Build history of the part. All positions in model axes, mm. Face numbers are marked on the shaded views. A direction names the side the tool comes from. Give positions to 0.01 mm unless a question says otherwise; leave off trailing zeros. Order: outer loops, then holes, each group sorted by start corner. A loop starts at its lowest first (then second) coordinate and runs counter-clockwise, first axis right, second up. Notation, with made-up numbers: (24, 44) -> (53, 44) arc R15 cw to (53, 65) -> close; hole circle Ø10 at (53, 45). An arc over 180 degrees is marked (long way). One line per item, written item: value. Start each with the question number.
(1) Pin check, flat tip, straight feed: pin 1 (2.5 mm diameter, centred on x = 10, z = 21, fed in from +Y). Stop position of the tip, or through.
(2) Two-plate mould, pull along X, no slides. Class the marked faces 1, 2, 3 and 4: +X half, -X half, draft (parallel to the pull), parting line (faces both ways), or undercut.
(3) Saw through at C-C on y = -10.25. Give the cut face in (x, z), plus the area to 3 significant figures.
(4) Saw through at A-A on y = -26.5. Give the cut face in (x, z), plus the area to 3 significant figures.
(5) Saw through at B-B on x = -4. Give the cut face in (y, z).
(6) Probe line 1 (Z direction, x = 13, y = -20.25); line 2 (Z direction, x = -8, y = -2.25); line 3 (Y direction, x = 16, z = 17.75). List the from-to ranges inside material, lowest first.
(7) Which spindle directions (+Z, -Z, +X, -X, +Y, -Y) get a long thin tool onto all of the face, cutting with end or side? Do the marked faces 5, 6 and 7. Say none if no direction does.
(8) Saw through at D-D on z = 22.25. Give the cut face in (x, y).
```python
from build123d import *

# Parameters (mm, degrees)
BOSS_EXTRUDE1_DEPTH         = 20.5
FILLET1_R                   = 2
M6_TAPPED_HOLE1_D           = 5
M6_TAPPED_HOLE1_DEPTH       = 17
M6_TAPPED_HOLE1_CSINK_D     = 6.05
M6_TAPPED_HOLE1_CSINK_ANGLE = 90
M6_TAPPED_HOLE1_TIP         = 1.502151548
FILLET2_R                   = 2


with BuildPart() as part:
    # Sketch1 → Boss-Extrude1 (new, symmetric)
    with BuildSketch(Plane(origin=(0, 0, 0), x_dir=(0, 0, -1), z_dir=(1, 0, 0))):
        with BuildLine():
            Line((-10, 0), (0, 0))
            Line((0, 0), (0, -30))
            Line((0, -30), (-26, -30))
            Line((-26, -30), (-26, -15))
            Line((-26, -15), (-16.32121885, -15))
            Line((-16.32121885, -15), (-12.897777479, -2.223542865))
            ThreePointArc((-12.897777479, -2.223542865), (-11.826284287, -0.619939979), (-10, 0))
        make_face()
    extrude(amount=BOSS_EXTRUDE1_DEPTH, both=True)

    # Fillet1
    fillet1_edges = [part.edges().sort_by_distance(p)[0] for p in [
        (20.5, -22.5, 26),
        (20.5, -15, 0),
        (-20.5, -15, 0),
        (-20.5, -22.5, 26),
    ]]
    fillet(fillet1_edges, radius=FILLET1_R)

    # M6 Tapped Hole1
    with Locations(Plane(origin=(0, -30, 0), x_dir=(-1, 0, 0), z_dir=(0, -1, 0))):
        with Locations((-13, -7.5), (13, -7.5)):
            CounterSinkHole(M6_TAPPED_HOLE1_D / 2, M6_TAPPED_HOLE1_CSINK_D / 2, depth=M6_TAPPED_HOLE1_DEPTH, counter_sink_angle=M6_TAPPED_HOLE1_CSINK_ANGLE)
            with Locations((0, 0, -(M6_TAPPED_HOLE1_DEPTH + M6_TAPPED_HOLE1_TIP / 2))):  # 118° drill point
                Cone(0, M6_TAPPED_HOLE1_D / 2, M6_TAPPED_HOLE1_TIP, mode=Mode.SUBTRACT)

    # Fillet2
    fillet2_edges = [part.edges().sort_by_distance(p)[0] for p in [
        (0, -15, 16.32121885),
    ]]
    fillet(fillet2_edges, radius=FILLET2_R)


solid = part.part
```
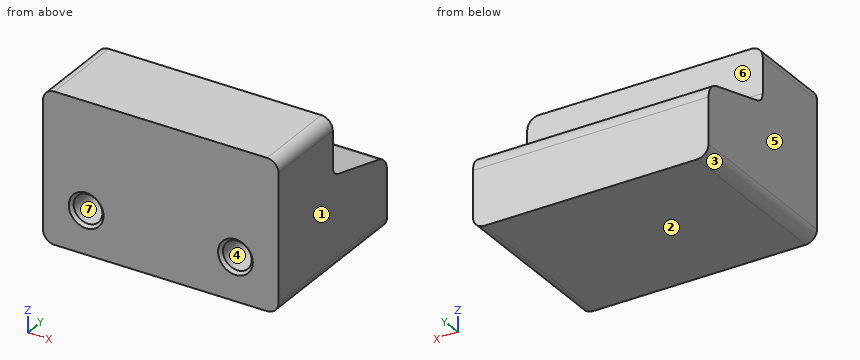
Results below:
1. pin 1: stops at y = -15
2. face 1: +X half
2. face 2: draft
2. face 3: -X half
2. face 4: undercut
3. outline: (-20.5, 2) arc R2 ccw to (-18.5, 0) -> (18.5, 0) arc R2 ccw to (20.5, 2) -> (20.5, 15.05) -> (-20.5, 15.05) -> close
3. area: 615 mm²
4. outline: (-20.5, 2) arc R2 ccw to (-18.5, 0) -> (18.5, 0) arc R2 ccw to (20.5, 2) -> (20.5, 24) arc R2 ccw to (18.5, 26) -> (-18.5, 26) arc R2 ccw to (-20.5, 24) -> close; hole circle Ø5 at (-13, 7.5); hole circle Ø5 at (13, 7.5)
4. area: 1,020 mm²
5. outline: (-30, 0) -> (0, 0) -> (0, 10) arc R3 ccw to (-2.22, 12.9) -> (-13.52, 15.92) arc R2 cw to (-15, 17.86) -> (-15, 26) -> (-30, 26) -> close
6. line 1: z = 0 to 5, 10 to 26
6. line 2: z = 0 to 12.9
6. line 3: y = -30 to -15
7. face 5: +Z, -Z, -X, +Y, -Y
7. face 6: +Z, +X, -X, +Y
7. face 7: -Y
8. outline: (-20.5, -30) -> (20.5, -30) -> (20.5, -15) -> (-20.5, -15) -> close
